The figure shows three views and two pictorial views of one solid part (mm, origin at its lowest corner). Answer the questions. A direction names the side the tool comes from. Round coordinates to 2 decimals unless told otherwise and drop trailing zeros. Write each loop counter-clockwise with the first axis right and the second up, starting at its lowest first coordinate (ties: lowest second). Pieces come first, ordered by that corner, then holes.
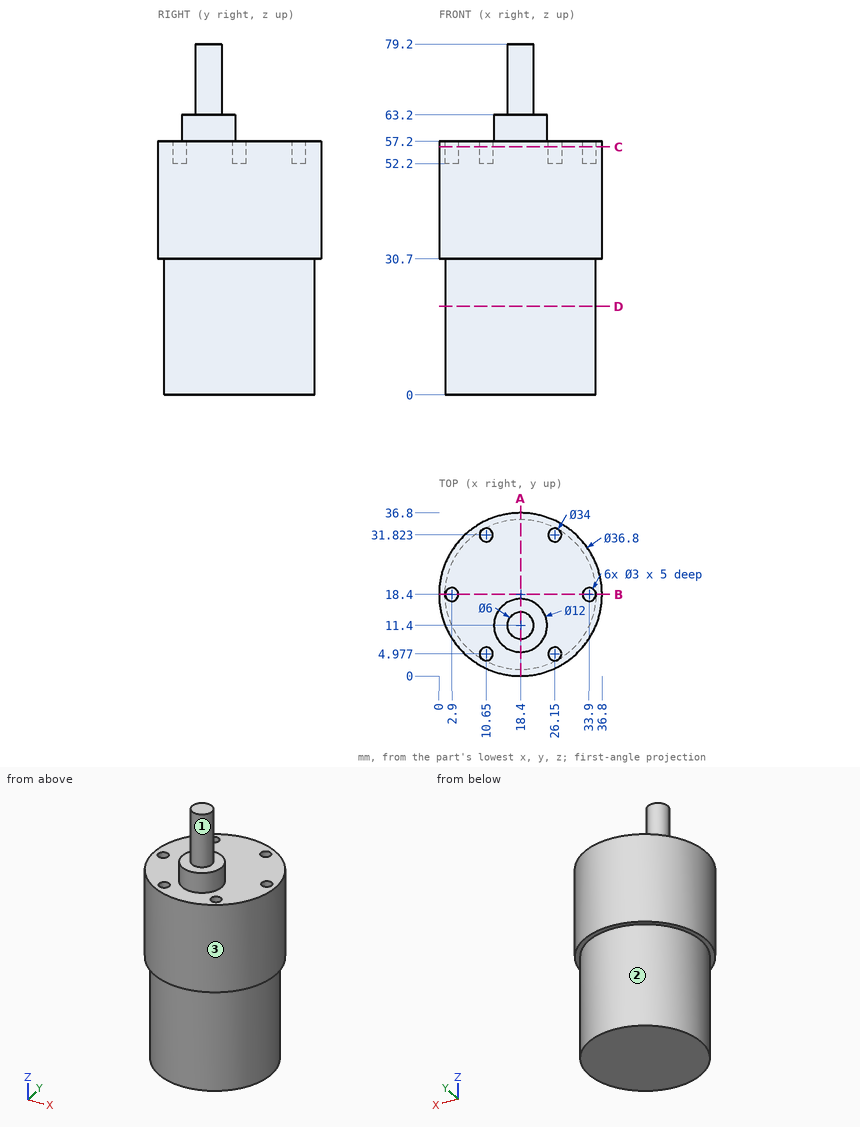
Q1. Section A-A (x = 18.4) is taken. Determine the outline of the cut face in (y, z).
Verdict:
outline: (0, 30.7) - (1.4, 30.7) - (1.4, 0) - (35.4, 0) - (35.4, 30.7) - (36.8, 30.7) - (36.8, 57.2) - (17.4, 57.2) - (17.4, 63.2) - (14.4, 63.2) - (14.4, 79.2) - (8.4, 79.2) - (8.4, 63.2) - (5.4, 63.2) - (5.4, 57.2) - (0, 57.2) - close
Q2. Section C-C (z = 56) is taken. Determine the outline of the cut face in (x, y).
Verdict:
outline: circle Ø36.8 at (18.4, 18.4); hole circle Ø3 at (2.9, 18.4); hole circle Ø3 at (10.65, 4.98); hole circle Ø3 at (10.65, 31.82); hole circle Ø3 at (26.15, 4.98); hole circle Ø3 at (26.15, 31.82); hole circle Ø3 at (33.9, 18.4)
Q3. Section B-B (y = 18.4) is taken. Determine the outline of the cut face in (x, z), then the cut area to 3 significant figures.
Verdict:
outline: (0, 30.7) - (1.4, 30.7) - (1.4, 0) - (35.4, 0) - (35.4, 30.7) - (36.8, 30.7) - (36.8, 57.2) - (35.4, 57.2) - (35.4, 52.2) - (32.4, 52.2) - (32.4, 57.2) - (4.4, 57.2) - (4.4, 52.2) - (1.4, 52.2) - (1.4, 57.2) - (0, 57.2) - close
area: 1,990 mm2
Q4. Straight lines are drawn through the part: probe 1 along Y at (x, z) = (26.15, 54.3); probe 2 along Z at (x, y) = (27.5, 2.5); probe 3 along Z at (x, y) = (30, 25.5). For each, find the intervals that lie inside material, in ascending order.
Verdict:
probe 1: y = 1.71 to 3.48, 6.48 to 30.32, 33.32 to 35.09
probe 2: z = 30.7 to 57.2
probe 3: z = 0 to 57.2
Q5. Section D-D (z = 20) is taken. Determine the outline of the cut face in (x, y), then the cut area to 3 significant figures.
Verdict:
outline: circle Ø34 at (18.4, 18.4)
area: 908 mm2
Q6. Flat-ended cylindrical pins translate along their axes: pin 1 Ø2 at (x, z) = (32, 40) entering from -Y; pin 2 Ø1.5 at (x, y) = (10, 4.5) entering from +Z; pin 3 Ø1.5 at (x, y) = (34, 19) entering from +Z; pin 4 Ø2.5 at (x, y) = (10.65, 4.98) entering from -Z. Find the tip coordinate at first contact, or state that the pin passes through.
Verdict:
pin 1: stops at y = 4.99
pin 2: stops at z = 57.2
pin 3: stops at z = 52.2
pin 4: stops at z = 0
Q7. Which of the six approach directions +Z, -Z, +X, -X, +Y, -Y give full straight-line access (tool end or side, diameter ignored) to the marked faces 1, 2 and 3?
Verdict:
face 1: +Z
face 2: -Z
face 3: +Z, -Z
